```python
from build123d import *

# Parameters (mm, degrees)
SKETCH1_W          = 5.5
SKETCH1_H          = 7
BASE_FLANGE1_DEPTH = 0.5
EDGE_FLANGE1_DEPTH = 7
EDGE_FLANGE2_DEPTH = 7
FILLET1_R          = 4
SKETCH12_R         = 2
CUT_EXTRUDE1_DEPTH = 16.880893326
SKETCH13_R         = 2
CUT_EXTRUDE2_DEPTH = 18.75106584


# Sheet-metal steps are written as plain solids
with BuildPart() as part:
    # Sketch1 → Base-Flange1 (new body)
    with BuildSketch(Plane(origin=(0, 0, 0), x_dir=(1, 0, 0), z_dir=(0, 1, 0))):
        Rectangle(SKETCH1_W, SKETCH1_H)
    extrude(amount=BASE_FLANGE1_DEPTH)

    # Edge-Flange1 section (across the edge) → Edge-Flange1 (add)
    with BuildSketch(Plane(origin=(3.4866, 0.5, 3.5), x_dir=(-1, 0, 0), z_dir=(0, 0, -1))):
        with BuildLine():
            Line((-0.5, 0.7366), (-0.5, 15))
            Line((-0.5, 15), (0, 15))
            Line((0, 15), (0, 0.7366))
            ThreePointArc((0, 0.7366), (0.215745145, 0.215745145), (0.7366, 0))
            Line((0.7366, 0), (0.7366, -0.5))
            ThreePointArc((0.7366, -0.5), (-0.137808246, -0.137808246), (-0.5, 0.7366))
        make_face()
    extrude(amount=EDGE_FLANGE1_DEPTH)

    # Edge-Flange2 section (across the edge) → Edge-Flange2 (add)
    with BuildSketch(Plane(origin=(-3.4866, 0.5, -3.5), x_dir=(1, 0, 0), z_dir=(0, 0, 1))):
        with BuildLine():
            Line((-0.5, 0.7366), (-0.5, 15))
            Line((-0.5, 15), (0, 15))
            Line((0, 15), (0, 0.7366))
            ThreePointArc((0, 0.7366), (0.215745145, 0.215745145), (0.7366, 0))
            Line((0.7366, 0), (0.7366, -0.5))
            ThreePointArc((0.7366, -0.5), (-0.137808246, -0.137808246), (-0.5, 0.7366))
        make_face()
    extrude(amount=EDGE_FLANGE2_DEPTH)

    # Fillet1
    # the kernel refuses this fillet: 4 mm, written as the material it takes off along each edge
    with BuildSketch(Plane(origin=(13.9866, 15.5, -3.5), x_dir=(0, -1, 0), z_dir=(-1, 0, 0)), Plane(origin=(13.9866, 15.5, 3.5), x_dir=(0, 0, -1), z_dir=(-1, 0, 0))) as fillet1_piece_1:
        with BuildLine():
            CenterArc((FILLET1_R, FILLET1_R), FILLET1_R, 180, 90)
            Line((0, FILLET1_R), (0, 0))
            Line((0, 0), (FILLET1_R, 0))
        make_face()
    extrude(amount=20.5, mode=Mode.SUBTRACT)
    with BuildSketch(Plane(origin=(-13.9866, 15.5, -3.5), x_dir=(0, -1, 0), z_dir=(1, 0, 0)), Plane(origin=(-13.9866, 15.5, 3.5), x_dir=(0, 0, -1), z_dir=(1, 0, 0))) as fillet1_piece_2:
        with BuildLine():
            CenterArc((FILLET1_R, -FILLET1_R), FILLET1_R, 90, 90)
            Line((0, -FILLET1_R), (0, 0))
            Line((0, 0), (FILLET1_R, 0))
        make_face()
    extrude(amount=20.5, mode=Mode.SUBTRACT)

    # Sketch12 → Cut-Extrude1 (cut, through all)
    with BuildSketch(Plane(origin=(0, 0.5, 0), x_dir=(1, 0, 0), z_dir=(0, 1, 0))):
        with Locations(Location((0, 0, 0), (0, 0, 270))):
            Circle(SKETCH12_R)
    extrude(amount=-CUT_EXTRUDE1_DEPTH, mode=Mode.SUBTRACT)

    # Sketch13 → Cut-Extrude2 (cut, through all)
    with BuildSketch(Plane(origin=(3.9866, 0, 0), x_dir=(0, 0, -1), z_dir=(1, 0, 0))):
        with Locations(Location((0, 11.678062377, 0), (0, 0, 90))):
            Circle(SKETCH13_R)
    extrude(amount=-CUT_EXTRUDE2_DEPTH, mode=Mode.SUBTRACT)


solid = part.part
```
Can you work these out from the model? Positions are in its coordinate system, mm. A direction names the side the tool comes from. Give positions to 0.01 mm unless a question says otherwise; leave off trailing zeros. Write each loop counter-clockwise with the first axis right and the second up, starting at its lowest first coordinate (ties: lowest second). Pieces come first, ordered by that corner, then holes. Notation, with made-up numbers: (-15.75, 7) - (6.25, 7) arc R13 ccw to (6.25, 25) - close; hole circle Ø1 at (73, 62). An arc over 180 degrees is marked (long way). Write item = value, one per line. Start each with the question number.
1. Imagine slicing it at B-B (x = 0.5). Please give me the cut outline in (y, z), and give its area (3 significant figures).
2. Imagine slicing it at D-D (y = 12). Please give me the cut outline in (x, z).
3. On a 3-axis mill with a long thin cutter (end or side, diameter ignored), from which of +Z, -Z, +X, -X, +Y, -Y can I reach the whole of each face in a straight line? I mean faces 1 (the face through (-3.487, 7, 0)), 2 (the face through (-2, 0, -1)). Say none if no direction works.
4. Please list where these lines run through material, in increasing order: line 1 (X direction, y = 5.5, z = -2.5); line 2 (X direction, y = 0.25, z = 0); line 3 (Y direction, x = 2.25, z = 2.5).
5. Imagine slicing it at C-C (z = 1.75). Please give me the cut outline in (x, y).
6. Imagine slicing it at A-A (y = 6). Please give me the cut outline in (x, z).
7. Thinking about a two-plate mould opening in Y: for faces 3 (the face through (3.74, 13.526, -0.766)), 4 (the face through (-3.61, 0.35, -0.05)), 5 (the face through (-3.733, 13.526, -0.766)), 6 (the face through (-3.987, 7, 0)), which applies, released by +Y, released by -Y, zero draft, split by the parting line, or undercut?
Worked answers:
q1.outline = (0, -3.5) - (0.5, -3.5) - (0.5, -1.94) - (0, -1.94) - close; (0, 1.94) - (0.5, 1.94) - (0.5, 3.5) - (0, 3.5) - close
q1.area = 1.56 mm2
q2.outline = (-3.99, -3.47) - (-3.49, -3.47) - (-3.49, -1.97) - (-3.99, -1.97) - close; (-3.99, 1.97) - (-3.49, 1.97) - (-3.49, 3.47) - (-3.99, 3.47) - close; (3.49, -3.47) - (3.99, -3.47) - (3.99, -1.97) - (3.49, -1.97) - close; (3.49, 1.97) - (3.99, 1.97) - (3.99, 3.47) - (3.49, 3.47) - close
q3.face_1 = +Z, -Z, +Y
q3.face_2 = +Z, -Z, +X, -X, -Y
q4.line_1 = -3.99 to -3.49, 3.49 to 3.99
q4.line_2 = -3.5 to -2, 2 to 3.5
q4.line_3 = 0 to 0.5
q5.outline = (-3.99, 1.24) arc R1.24 ccw to (-2.75, 0) - (-0.97, 0) - (-0.97, 0.5) - (-2.75, 0.5) arc R0.74 cw to (-3.49, 1.24) - (-3.49, 10.71) - (-3.99, 10.71) - close; (-3.99, 12.65) - (-3.49, 12.65) - (-3.49, 14.81) - (-3.99, 14.81) - close; (0.97, 0) - (2.75, 0) arc R1.24 ccw to (3.99, 1.24) - (3.99, 10.71) - (3.49, 10.71) - (3.49, 1.24) arc R0.74 cw to (2.75, 0.5) - (0.97, 0.5) - close; (3.49, 12.65) - (3.99, 12.65) - (3.99, 14.81) - (3.49, 14.81) - close
q6.outline = (-3.99, -3.5) - (-3.49, -3.5) - (-3.49, 3.5) - (-3.99, 3.5) - close; (3.49, -3.5) - (3.99, -3.5) - (3.99, 3.5) - (3.49, 3.5) - close
q7.face_3 = undercut
q7.face_4 = released by -Y
q7.face_5 = undercut
q7.face_6 = zero draft
